The listing builds one solid part. Answer for the finished solid, in the listing's coordinates (mm). Face numbers are marked on the shaded views. A direction names the side the tool comes from. Round coordinates to 2 decimals unless told otherwise and drop trailing zeros. Write each loop counter-clockwise with the first axis right and the second up, starting at its lowest first coordinate (ties: lowest second). Pieces come first, ordered by that corner, then holes.
Item 1: For a pull along X with two mould halves and no side action, classify the marked faces 1 and 2 as +X half, -X half, draft (parallel to the pull), parting line (faces both ways), or undercut.
Item 2: Find section A-A on z = 0. Give the vertices of the cut face in (x, y).
Item 3: A tool of negligible diameter and unlimited length cuts with its end or side. For the marked faces 3, 4, 5 and 6, from which of +Z, -Z, +X, -X, +Y, -Y can it reach the whole face along a straight path? Write none if from no direction.
Item 4: Each of these flat-tipped pins is pushed along its axis until it touches: pin 1 (5 mm diameter, centred on y = 9, z = 13.5, fed in from -X); pin 2 (1 mm diameter, centred on y = 15, z = -20, fed in from -X); pin 3 (4 mm diameter, centred on y = 9, z = -22, fed in from +X); pin 4 (4 mm diameter, centred on x = 0, z = 0, fed in from +Y) (3 decimals). Where does it stop, or does it pass through?
Item 5: Find the intervals of material crossed by probe 1 along X at (y, z) = (18, 0); probe 2 along X at (y, z) = (4.5, -26.5); probe 3 along Z at (x, y) = (20.5, 17.5), in increasing order.
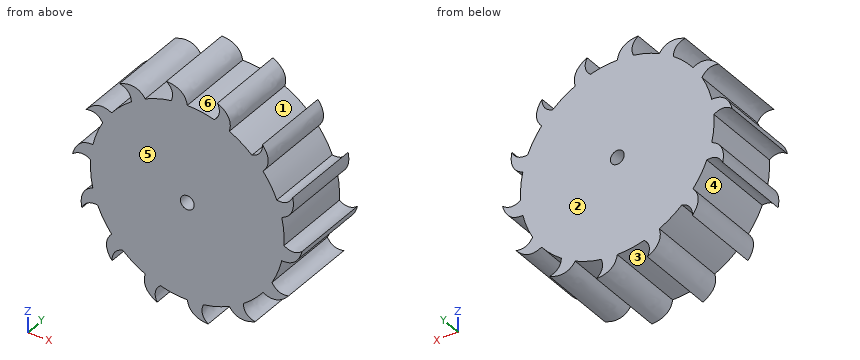
```python
from build123d import *

# Parameters (mm, degrees)
SKETCH1_R           = 30
BOSS_EXTRUDE1_DEPTH = 25
SKETCH2_R           = 2.15
CUT_EXTRUDE1_DEPTH  = 26
BOSS_EXTRUDE2_DEPTH = 25
CIRPATTERN1_COUNT   = 14


with BuildPart() as part:
    # Sketch1 → Boss-Extrude1 (new body)
    with BuildSketch(Plane(origin=(0, 0, 0), x_dir=(1, 0, 0), z_dir=(0, 1, 0))):
        Circle(SKETCH1_R)
    extrude(amount=BOSS_EXTRUDE1_DEPTH)

    # Sketch2 → Cut-Extrude1 (cut, through all)
    with BuildSketch(Plane(origin=(0, 25, 0), x_dir=(1, 0, 0), z_dir=(0, 1, 0))):
        Circle(SKETCH2_R)
    extrude(amount=-CUT_EXTRUDE1_DEPTH, mode=Mode.SUBTRACT)

    # Sketch3 → Boss-Extrude2 (add, through all)
    with BuildSketch(Plane(origin=(0, 25, 0), x_dir=(1, 0, 0), z_dir=(0, 1, 0))):
        with BuildLine():
            Line((0, 30), (3.378956964, 26.809860285))
            Line((3.378956964, 26.809860285), (4.977675541, 29.584163774))
            add(Edge.make_bspline(
                [(6.463090103, 34.958464686), (3.678095749, 32.81046922), (4.977675541, 29.584163774)],
                knots=[0, 0, 0, 1, 1, 1], degree=2))
            add(Edge.make_bspline(
                [(0, 30), (0.774451362, 34.774618744), (6.463090103, 34.958464686)],
                knots=[0, 0, 0, 1, 1, 1], degree=2))
        make_face()
    boss_extrude2 = extrude(amount=-BOSS_EXTRUDE2_DEPTH)

    # CirPattern1: Boss-Extrude2 ×14 about axis
    cirpattern1_axis = Axis((0, 0, 0), (0, 1, 0))
    for i in range(1, CIRPATTERN1_COUNT):
        add(boss_extrude2.rotate(cirpattern1_axis, i * 360 / CIRPATTERN1_COUNT))


solid = part.part
```
Check values:
1. face 1: undercut
1. face 2: draft
2. outline: (-30, 0) - (-2.15, 0) - (-2.15, 25) - (-30, 25) - close; (2.15, 0) - (30, 0) - (30, 25) - (2.15, 25) - close
3. face 3: -Z, +Y, -Y
3. face 4: +Y, -Y
3. face 5: +Z, -Z, +X, -X, -Y
3. face 6: +Z, +Y, -Y
4. pin 1: stops at x = -27.91
4. pin 2: stops at x = -24.64
4. pin 3: stops at x = 22.36
4. pin 4: passes through
5. probe 1: x = -30 to -2.15, 2.15 to 30
5. probe 2: x = -23.55 to -23.3, -14.06 to 17.83
5. probe 3: z = -28.9 to -28.57, -21.9 to 22.5
